```python
from build123d import *

# Parameters (mm, degrees)
BOSS_EXTRUDE1_DEPTH     = 175
SKETCH2_R               = 1.9
CUT_EXTRUDE1_DEPTH      = 176.775126352
CUT_EXTRUDE2_DEPTH      = 176.775126352
CUT_EXTRUDE2_DEPTH_BACK = 176.775126352
SKETCH3_R               = 1.9


with BuildPart() as part:
    # Sketch1 → Boss-Extrude1 (new body)
    with BuildSketch(Plane.XY):
        Polygon((0, 0), (11.68185891, 0), (10.66371782, 11.63740591), (-1.01814109, 11.63740591), align=None)
    extrude(amount=BOSS_EXTRUDE1_DEPTH)

    # Sketch2 → Cut-Extrude1 (cut, through all)
    with BuildSketch(Plane(origin=(0, 0, 0), x_dir=(1, 0, 0), z_dir=(0, 1, 0))):
        with Locations(Location((5.33185891, -8, 0), (0, 0, 270))):
            Circle(SKETCH2_R)
        with Locations(Location((5.33185891, -167, 0), (0, 0, 270))):
            Circle(SKETCH2_R)
    extrude(amount=CUT_EXTRUDE1_DEPTH, mode=Mode.SUBTRACT)

    # Sketch3 → Cut-Extrude2 (cut, two sides: drawn at the far end of the back side and taken through both)
    with BuildSketch(Plane(origin=(11.593122067, 1.014266756, 0), x_dir=(0, 0, -1), z_dir=(0.9961946980917453, 0.08715574274766183, 0)).offset(-CUT_EXTRUDE2_DEPTH_BACK)):
        with Locations(Location((-160, 5.33185891, 0), (0, 0, 90))):
            Circle(SKETCH3_R)
        with Locations(Location((-15, 5.33185891, 0), (0, 0, 90))):
            Circle(SKETCH3_R)
    extrude(amount=CUT_EXTRUDE2_DEPTH + CUT_EXTRUDE2_DEPTH_BACK, mode=Mode.SUBTRACT)


solid = part.part
```
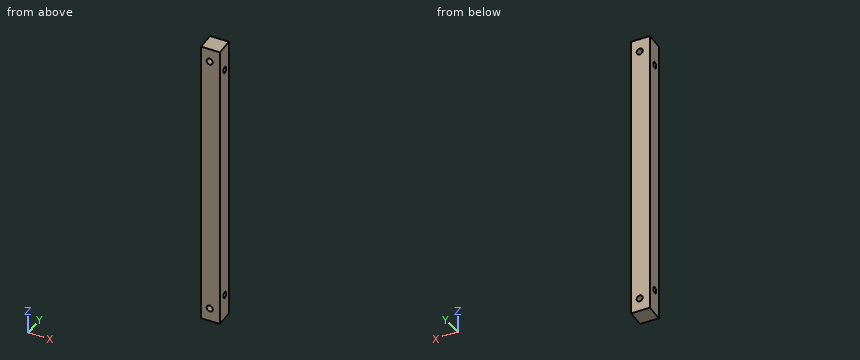
For this review, take the finished solid that the model builds, in its own axes (mm). Give positions to 0.01 mm unless a question says otherwise; leave off trailing zeros. Write each loop counter-clockwise with the first axis right and the second up, starting at its lowest first coordinate (ties: lowest second). Pieces come first, ordered by that corner, then holes.
Item 1: Take a section at C-C (z = 32). Give the boundary of the cut face in (x, y), and give its area (3 significant figures).
Item 2: Take a section at A-A (z = 167). Give the boundary of the cut face in (x, y).
Item 3: Insertion check: P1, Ø3, axis at y = 6.5, z = 22, coming from the -X side; P2, Ø1.5, axis at y = 8.5, z = 130.5, coming from the -X side. Each pin has a flat end and moves straight along its axis. Give the tip position at first contact, or say it passes through.
Item 4: Wall thickness on probe 1 along Z at (x, y) = (7.5, 5.75); probe 2 along Z at (x, y) = (5.25, 6); probe 3 along Z at (x, y) = (5.75, 2.75): over which ranges is each line inside the solid? List them lowest first.
Item 5: Take a section at B-B (y = 5.5). Give the number of separate pieces and of enclosed holes in the cut face, and give its area (3 significant figures).
Established:
1. outline: (-1.02, 11.64) - (0, 0) - (11.68, 0) - (10.66, 11.64) - close
1. area: 136 mm2
2. outline: (-1.02, 11.64) - (0, 0) - (3.43, 0) - (3.43, 11.64) - close; (7.23, 0) - (11.68, 0) - (10.66, 11.64) - (7.23, 11.64) - close
3. P1: stops at x = -0.7
3. P2: stops at x = -0.81
4. probe 1: z = 0 to 13.12, 16.88 to 158.12, 161.88 to 175
4. probe 2: z = 0 to 6.1, 9.9 to 13.11, 16.89 to 158.11, 161.89 to 165.1, 168.9 to 175
4. probe 3: z = 0 to 6.15, 9.85 to 165.15, 168.85 to 175
5. separate pieces: 3
5. enclosed holes: 2
5. area: 1,940 mm2
